Part model, mm, in its own coordinate system. A direction names the side the tool comes from. Coordinates: 2 decimals unless noted, no trailing zeros. Write each loop counter-clockwise with the first axis right and the second up, starting at its lowest first coordinate (ties: lowest second). Pieces come first, ordered by that corner, then holes. Notation, with made-up numbers: (-25, 23.5) -> (34, 23.5) arc R18 cw to (34, 57.5) -> close; hole circle Ø9 at (-34.5, 54). An arc over 180 degrees is marked (long way). One line per question, with ' | ' between items. Start each with the question number.
Item 1: Saw through at B-B (x = -3.5). List the corners of the cut face in (y, z), and give its area (3 significant figures).
Item 2: 3-axis set-ups, long thin cutter, end or side, ignore diameter. For faces 1 (the flat face through (47, 3.175, -4)), 2 (the cylindrical face through (3.67, 4.6, -9.39)), 3 (the flat face through (-22, 6, 0)), 4 (the cylindrical face through (63.61, 1.57, -15.38)), 5 (the flat face through (64.3, 2, 1)): which of +Z, -Z, +X, -X, +Y, -Y reach the whole face in a straight line?
Item 3: Saw through at A-A (z = 14). List the corners of the cut face in (x, y) (3 decimals).
Item 4: Two-plate mould, pull along X, no slides. Class faces 6 (the flat face through (-28, 4.762, -9)), 7 (the cylindrical face through (16.633, 0.154, -9.392)), 8 (the cylindrical face through (63.39, 1.61, 18.1)), 9 (the cylindrical face through (-61.913, 5.674, -9.392)): pulls with the +X half, pulls with the -X half, needs draft (parallel to the pull), parting line crosses it, or undercut.
Item 5: Pin check, flat tips, straight feed: pin 1 (8.5 mm diameter, centred on x = 51.6, z = -9.52, fed in from +Y) (3 decimals); pin 2 (4 mm diameter, centred on x = -21, y = 5.5, fed in from +Z); pin 3 (3 mm diameter, centred on x = -12, z = -10.5, fed in from -Y). Stop position of each tip, or through.
Item 6: Probe probe 1 along Y at (x, z) = (42, -5.5) (3 decimals); probe 2 along Z at (x, y) = (8, 3.25); probe 3 along Y at (x, z) = (-1.5, -9). List the from-to ranges inside material, lowest first. Write a range as [from, to].
from build123d import *

# Parameters (mm, degrees)
SKETCH2_W               = 128.6002
SKETCH2_H               = 38.1
BOSS_EXTRUDE1_DEPTH     = 7.9375
CUT_EXTRUDE1_DEPTH      = 7.9375
CUT_EXTRUDE3_DEPTH      = 7.9375
FILLET3_R               = 3.175
SKETCH6_R               = 3.175
CUT_EXTRUDE4_DEPTH      = 7.9375
CUT_EXTRUDE8_DEPTH      = 76.160606479
CUT_EXTRUDE8_DEPTH_BACK = 76.160606479
SKETCH12_W              = 13.089840981
SKETCH12_H              = 4.7625


with BuildPart() as part:
    # Sketch2 → Boss-Extrude1 (new body)
    with BuildSketch(Plane(origin=(0, 0, 0), x_dir=(1, 0, 0), z_dir=(0, 1, 0))):
        Rectangle(SKETCH2_W, SKETCH2_H)
    extrude(amount=BOSS_EXTRUDE1_DEPTH)

    # Sketch4 → Cut-Extrude1 (cut)
    with BuildSketch(Plane(origin=(0, 7.9375, 0), x_dir=(1, 0, 0), z_dir=(0, 1, 0))):
        Polygon((64.3001, 19.05), (51.6001, 19.05), (64.3001, 15.883534364), align=None)
    extrude(amount=-CUT_EXTRUDE1_DEPTH, mode=Mode.SUBTRACT)

    # Sketch5 → Cut-Extrude3 (cut)
    with BuildSketch(Plane(origin=(0, 7.9375, 0), x_dir=(1, 0, 0), z_dir=(0, 1, 0))):
        with BuildLine():
            Line((-64.3001, 0), (21.860482552, 0))
            ThreePointArc((21.860482552, 0), (27.332932171, -1.088537909), (31.972250944, -4.188431608))
            Line((31.972250944, -4.188431608), (44.505259668, -16.721440332))
            ThreePointArc((44.505259668, -16.721440332), (47.084490176, -18.444827059), (50.1269, -19.05))
            Line((50.1269, -19.05), (-64.3001, -19.05))
            Line((-64.3001, -19.05), (-64.3001, 0))
        make_face()
    extrude(amount=-CUT_EXTRUDE3_DEPTH, mode=Mode.SUBTRACT)

    # Fillet3
    fillet3_edges = [part.edges().sort_by_distance(p)[0] for p in [
        (64.3001, 3.96875, -15.883534364),
        (51.6001, 3.96875, -19.05),
        (64.3001, 3.96875, 19.05),
    ]]
    fillet(fillet3_edges, radius=FILLET3_R)

    # Sketch6 → Cut-Extrude4 (cut)
    with BuildSketch(Plane(origin=(0, 7.9375, 0), x_dir=(1, 0, 0), z_dir=(0, 1, 0))):
        with Locations(Location((51.6001, 9.525, 0), (0, 0, 270))):
            Circle(SKETCH6_R)
        with Locations(Location((51.6001, -12.7, 0), (0, 0, 270))):
            Circle(SKETCH6_R)
    extrude(amount=-CUT_EXTRUDE4_DEPTH, mode=Mode.SUBTRACT)

    # Sketch12 → Cut-Extrude8 (cut, two sides: drawn at the far end of the back side and taken through both)
    with BuildSketch(Plane(origin=(0, 0, -19.05), x_dir=(-1, 0, 0), z_dir=(0, 0, -1)).offset(-CUT_EXTRUDE8_DEPTH_BACK)):
        with BuildLine():
            Line((-10.637677607, 5.644085453), (-6.179942499, 7.266568345))
            ThreePointArc((-6.179942499, 7.266568345), (-4.306770706, 7.768483214), (-2.3749, 7.9375))
            Line((-2.3749, 7.9375), (-51.210259019, 7.9375))
            Line((-51.210259019, 7.9375), (-51.210259019, 3.175))
            Line((-51.210259019, 3.175), (-24.615767874, 3.175))
            Line((-24.615767874, 3.175), (-18.823268898, 3.175))
            ThreePointArc((-18.823268898, 3.175), (-17.442731156, 3.295781402), (-16.104140354, 3.654455726))
            Line((-16.104140354, 3.654455726), (-10.637677607, 5.644085453))
        make_face()
        with Locations((-57.75517951, 5.55625)):
            Rectangle(SKETCH12_W, SKETCH12_H)
        with BuildLine():
            ThreePointArc((56.3626, 7.9375), (61.975260076, 5.612660076), (64.3001, 0))
            Line((64.3001, 0), (64.3001, 7.9375))
            Line((64.3001, 7.9375), (56.3626, 7.9375))
        make_face()
        with BuildLine():
            ThreePointArc((61.1251, 0), (59.730196045, 3.367596045), (56.3626, 4.7625))
            Line((56.3626, 4.7625), (-1.766638139, 4.7625))
            ThreePointArc((-1.766638139, 4.7625), (-3.698508845, 4.593483214), (-5.571680637, 4.091568345))
            Line((-5.571680637, 4.091568345), (-12.417211155, 1.599998998))
            Line((-12.417211155, 1.599998998), (-15.530771457, 0.466755726))
            ThreePointArc((-15.530771457, 0.466755726), (-16.648641249, 0.150225095), (-17.800707625, 0))
            Line((-17.800707625, 0), (48.4251, 0))
            Line((48.4251, 0), (51.6001, 0))
            Line((51.6001, 0), (61.1251, 0))
        make_face()
    extrude(amount=CUT_EXTRUDE8_DEPTH + CUT_EXTRUDE8_DEPTH_BACK, mode=Mode.SUBTRACT)


solid = part.part
From the geometry:
1) outline: (4.76, -19.05) -> (7.94, -19.05) -> (7.94, 0) -> (4.76, 0) -> close | area: 60.5 mm2
2) face 1: +Z, -Z, +X, +Y | face 2: +Z, -Z, -Y | face 3: +Z, -X, +Y, -Y | face 4: -Z, +X, +Y, -Y | face 5: +Z, -Z, +X, +Y, -Y
3) outline: (41.784, 0) -> (48.703, 0) -> (48.703, 3.175) -> (41.784, 3.175) -> close; (54.497, 0) -> (64.3, 0) -> (64.3, 3.175) -> (54.497, 3.175) -> close
4) face 6: undercut | face 7: undercut | face 8: pulls with the +X half | face 9: pulls with the -X half
5) pin 1: y = 3.175 | pin 2: z = 0 | pin 3: y = 4.76
6) probe 1: [0, 3.175] | probe 2: [-19.05, 0] | probe 3: [4.76, 7.94]
